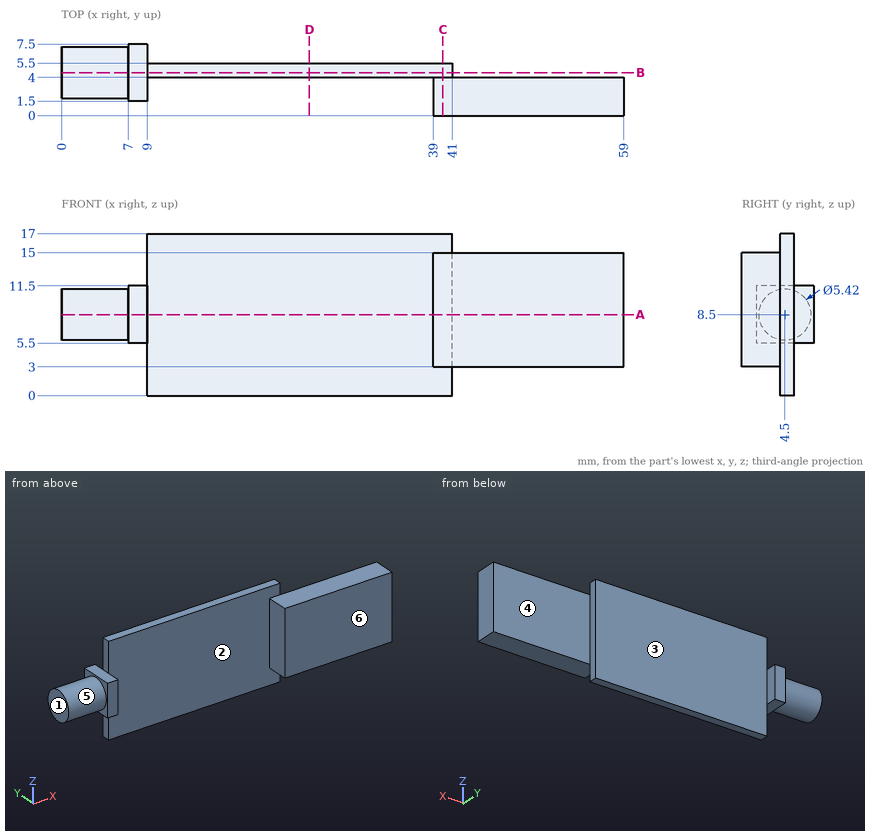
Print and shaded views of the part. All mm, measured from the part's lowest x, y and z. A direction names the side the tool comes from. Round coordinates to 2 decimals unless told otherwise and drop trailing zeros. Order: outer loops, then holes, each group sorted by start corner. A loop starts at its lowest first (then second) coordinate and runs counter-clockwise, first axis right, second up.
Q1. Wall check: L1, parallel to X at y = 2.75, z = 9.5; L2, parallel to X at y = 2.5, z = 6; L3, parallel to Y at x = 56, z = 8. Give the ranges that are in metal, low to high.
Q2. Which spindle directions (+Z, -Z, +X, -X, +Y, -Y) get a long thin tool onto all of the face, cutting with end or side? Do the marked faces 4, 5 and 6. Say none if no direction does.
Q3. Slice it at C-C (x = 40). Write the cut outline in (y, z), and give its area (3 significant figures).
Q4. Drop flat-ended pins along their axis: pin 1 (4 mm diameter, centred on y = 4.5, z = 9.5, fed in from -X); pin 2 (3.5 mm diameter, centred on x = 54, z = 6.5, fed in from +Y); pin 3 (0.6 mm diameter, centred on x = 8, y = 4, fed in from +Z); pin 4 (1.6 mm diameter, centred on x = 8, y = 4.5, fed in from -Z). Give the stop position or say it passes through.
Q5. Two-plate mould, pull along X, no slides. Class the marked faces 1, 2 and 3: pulls with the +X half, pulls with the -X half, needs draft (parallel to the pull), parting line crosses it, or undercut.
Q6. Slice it at B-B (y = 4.5). Write the cut outline in (x, z), and give its area (3 significant figures).
Q7. Slice it at A-A (z = 8.5). Write the cut outline in (x, y), and give its area (3 significant figures).
Q8. Slice it at D-D (x = 26). Write the cut outline in (y, z), and give its area (3 significant figures).
Results below:
1. L1: x = 0 to 9, 39 to 59
1. L2: x = 7 to 9, 39 to 59
1. L3: y = 0 to 4
2. face 4: +Z, -Z, +X, +Y
2. face 5: -X
2. face 6: +Z, -Z, +X, -X, -Y
3. outline: (0, 3) - (4, 3) - (4, 0) - (5.5, 0) - (5.5, 17) - (4, 17) - (4, 15) - (0, 15) - close
3. area: 73.5 mm2
4. pin 1: stops at x = 0
4. pin 2: stops at y = 4
4. pin 3: stops at z = 11.5
4. pin 4: stops at z = 5.5
5. face 1: pulls with the -X half
5. face 2: undercut
5. face 3: needs draft
6. outline: (0, 5.79) - (7, 5.79) - (7, 5.5) - (9, 5.5) - (9, 0) - (41, 0) - (41, 17) - (9, 17) - (9, 11.5) - (7, 11.5) - (7, 11.21) - (0, 11.21) - close
6. area: 594 mm2
7. outline: (0, 1.79) - (7, 1.79) - (7, 1.5) - (9, 1.5) - (9, 4) - (39, 4) - (39, 0) - (59, 0) - (59, 4) - (41, 4) - (41, 5.5) - (9, 5.5) - (9, 7.5) - (7, 7.5) - (7, 7.21) - (0, 7.21) - close
7. area: 178 mm2
8. outline: (4, 0) - (5.5, 0) - (5.5, 17) - (4, 17) - close
8. area: 25.5 mm2
